Check sheet for the modelled part. Datum: model origin and axes. Units: mm. Face numbers are marked on the shaded views. A direction names the side the tool comes from. Round coordinates to 2 decimals unless told otherwise and drop trailing zeros. Write each loop counter-clockwise with the first axis right and the second up, starting at its lowest first coordinate (ties: lowest second). Pieces come first, ordered by that corner, then holes. Notation, with made-up numbers: (88.25, -35.5) -> (128.25, -35.5) arc R31 ccw to (128.25, 3.5) -> close; hole circle Ø10 at (-11, 47). An arc over 180 degrees is marked (long way). One line per item, written item: value.
Autodesk Inventor part; units mm, degrees
ref_plane "YZ Plane" through (0, 0, 0) normal (1, 0, 0) x (0, 1, 0)
ref_plane "XZ Plane" through (0, 0, 0) normal (0, 1, 0) x (-1, 0, 0)
ref_plane "XY Plane" through (0, 0, 0) normal (0, 0, 1) x (1, 0, 0)
sketch "Sketch1" plane through (0, 0, 0) normal (0, 1, 0) x (-1, 0, 0)
  line L0 (25.9, 0) -> (-25.9, 0)
  line L1 (0, -25.9) -> (0, 25.9)
  circle A0 centre (0, 0) radius 18.5 construction
  circle A1 centre (0, 0) radius 13 construction
  dimension "d0" = 37
  dimension "d1" = 26
sketch "Sketch2" plane through (0, 0, 0) normal (0, 1, 0) x (-1, 0, 0)
  line L0 (77.7, 0) -> (-77.7, 0)
  line L1 (0, -33.3) -> (0, 70.3)
  line L2 (-55.5, 55.5) -> (-55.5, -18.5)
  line L3 (-55.5, -18.5) -> (55.5, -18.5)
  line L4 (55.5, -18.5) -> (55.5, 55.5)
  line L5 (-55.5, 55.5) -> (55.5, 55.5)
  circle A0 centre (0, 37) radius 18.5 construction
  point P0 (0, 0)
  dimension "d3" = 111
  dimension "d29" = 18.5
  dimension "d30" = 55.5
  dimension "d99" = 37
  dimension "d100" = 37
extrude "Extrusion1" add sketch "Sketch2" along normal blind 6
sketch "Sketch6" plane through (0, 0, 0) normal (0, 1, 0) x (-1, 0, 0)
  line L0 (55.5, -18.5) -> (-55.5, -18.5)
  line L1 (55.5, 55.5) -> (55.5, -18.5)
  line L2 (-55.5, -18.5) -> (55.5, -18.5)
  line L3 (55.5, -18.5) -> (55.5, 55.5)
  line L4 (-55.5, 55.5) -> (-55.5, -18.5)
  line L5 (84.7, 0) -> (-84.7, 0)
  line L6 (0, -36.3) -> (0, 70.8)
  arc A0 (-16, 0) -> (16, 0) centre (0, 0) ccw
  line L7 (16, 0) -> (16, 55.5)
  line L8 (55.5, 55.5) -> (-55.5, 55.5)
  line L9 (16, 55.5) -> (55.5, 55.5)
  line L10 (-16, 0) -> (-16, 55.5)
  line L11 (-16, 55.5) -> (-55.5, 55.5)
  point P0 (-17.3617, -21)
  dimension "d18" = 32
extrude "Extrusion5" [suppressed]
sketch "Sketch4" plane through (0, 0, 0) normal (0, 0, 1) x (1, 0, 0)
  line L0 (-18.5, 0) -> (18.5, 0)
  line L1 (18.5, 0) -> (18.5, -2)
  line L2 (18.5, -2) -> (-18.5, -2)
  line L3 (-18.5, -2) -> (-18.5, 0)
  line L4 (-25.9, 0) -> (25.9, 0)
  line L5 (0, -2.4) -> (0, 0.4)
  point P0 (0, 0)
  dimension "d10" = 37
  dimension "d11" = 2
extrude "Extrusion6" [suppressed]
sketch "Sketch5" plane through (0, 0, 0) normal (0, 1, 0) x (-1, 0, 0)
  circle A0 centre (0, 0) radius 18.5 construction
  circle A1 centre (0, 0) radius 18.5 construction
  line L0 (25.9, 0) -> (-25.9, 0)
  line L1 (0, -28.9) -> (0, 26.4)
  line L2 (-18.5, -21) -> (18.5, -21)
  line L3 (18.5, -21) -> (18.5, -18.5)
  line L4 (18.5, -18.5) -> (-18.5, -18.5)
  line L5 (-18.5, -18.5) -> (-18.5, -21)
  dimension "d25" = 37
  dimension "d26" = 21
extrude "Extrusion7" [suppressed]
sketch "Sketch7" plane through (0, 0, 0) normal (0, 0, 1) x (1, 0, 0)
  line L0 (-18.5, 0) -> (18.5, 0)
  line L1 (18.5, 0) -> (18.5, -2)
  line L2 (18.5, -2) -> (-18.5, -2)
  line L3 (-18.5, -2) -> (-18.5, 0)
  line L4 (55.5, 0) -> (-55.5, 0)
  line L5 (-84.7, 0) -> (84.7, 0)
  line L6 (0, -2.4) -> (0, 0.4)
  point P0 (-16, 0)
  point P1 (16, 0)
  dimension "d53" = 2
  dimension "d54" = 18.5
extrude "Extrusion8" [suppressed]
sketch "Sketch8" plane through (0, 0, 0) normal (0, 1, 0) x (-1, 0, 0)
  circle A0 centre (0, 0) radius 12.75
  dimension "d34" = 25.5
extrude "Extrusion9" add sketch "Sketch8" along normal blind 14
pattern_linear "Rectangular Pattern1" count 2 spacing 37 along (0, 0, 1) count 3 spacing 37 along (1, 0, 0) of "Extrusion9" second direction both ways yes
sketch "Sketch9" plane through (0, 6, 0) normal (0, 1, 0) x (1, 0, 0)
  circle A0 centre (0, 0) radius 13
  circle A1 centre (0, 0) radius 15
  dimension "d40" = 26
  dimension "d41" = 30
extrude "Extrusion10" [suppressed]
sketch "Sketch10" plane through (0, 5, 0) normal (0, 1, 0) x (1, 0, 0)
  arc A0 (16, 0) -> (-16, 0) centre (0, 0) ccw
  line L0 (1.5, -18) -> (-1.5, -18)
  line L1 (-29.4, 0) -> (29.4, 0)
  line L2 (0, 36.3) -> (0, -70.8)
  line L3 (1.5, -12) -> (-1.5, -12)
  line L4 (1.5, -12) -> (1.5, -18)
  line L5 (-1.5, -18) -> (-1.5, -12)
  dimension "d48" = 3
  dimension "d49" = 12
  dimension "d50" = 6
extrude "Extrusion11" [suppressed]
fillet "Fillet1" [suppressed]
sketch "Sketch11" plane through (0, 0, 0) normal (0, 1, 0) x (-1, 0, 0)
  line L0 (-60.5, -21) -> (60.5, -21)
  line L1 (60.5, -21) -> (60.5, -47)
  line L2 (60.5, -47) -> (-60.5, -47)
  line L3 (-60.5, -47) -> (-60.5, -21)
  line L4 (84.7, 0) -> (-84.7, 0)
  line L5 (0, -60.1) -> (0, 31.6)
  point P0 (0, 0)
  dimension "d57" = 26
  dimension "d58" = 21
  dimension "d59" = 121
extrude "Extrusion12" [suppressed]
sketch "Sketch12" plane through (0, 0, 0) normal (1, 0, 0) x (0, 1, 0)
  line L0 (6, 55.5) -> (6, -18.5)
  arc A0 (6, -16.5081) -> (5.7334, -47) centre (34, -32) ccw
  line L1 (-6.8, 0) -> (40.8, 0)
  line L2 (0, -67.5) -> (0, 76)
  line L3 (6, -16.5081) -> (6, -47)
  line L4 (6, -47) -> (5.7334, -47)
  line L5 (0, -47) -> (6, -47)
  point P0 (0, 0)
  point P1 (6, 48)
  dimension "d62" = 32
  dimension "d63" = 32
  dimension "d64" = 34
extrude "Extrusion13" [suppressed]
fillet "Fillet3" [suppressed]
sketch "Sketch13" plane through (0, 0, 0) normal (0, 1, 0) x (-1, 0, 0)
  line L0 (84.7, 0) -> (-84.7, 0)
  line L1 (0, -67.5) -> (0, 76)
  line L2 (55.5, 55.5) -> (55.5, -18.5)
  arc A0 (13.0815, 23.9185) -> (13.0815, 13.0815) centre (18.5, 18.5) ccw
  line L3 (-55.5, 55.5) -> (-55.5, -18.5)
  arc A1 (-13.0815, 13.0815) -> (-13.0815, 23.9185) centre (-18.5, 18.5) ccw
  line L4 (18.5, 37) -> (18.5, 0)
  line L5 (-18.5, 0) -> (-18.5, 37)
  line L6 (18.5, 37) -> (18.5, 55.5)
  line L7 (-55.5, 55.5) -> (55.5, 55.5)
  line L8 (-18.5, 55.5) -> (-18.5, 37)
  arc A2 (-9.2871, 53) -> (-13.0815, 23.9185) centre (0, 37) ccw
  arc A3 (13.0815, 23.9185) -> (9.2871, 53) centre (0, 37) ccw
  arc A4 (-13.0815, 13.0815) -> (-18.5, 0) centre (0, 0) ccw
  arc A5 (18.5, 0) -> (13.0815, 13.0815) centre (0, 0) ccw
  point P0 (60.5, -39.254)
  point P1 (-55.5, 48)
  point P2 (-60.5, -16.5081)
  point P3 (-60.5, -47)
  point P4 (55.5, -18.5)
  point P5 (-55.5, -18.5)
  dimension "d68" = 37
  dimension "d71" = 18.5
  dimension "d72" = 18.5
  dimension "d73" = 7.663
  dimension "d74" = 7.663
  dimension "d75" = 18.5
  dimension "d76" = 18.5
  dimension "d77" = 18.5
  dimension "d78" = 18.5
extrude "Extrusion14" [suppressed]
sketch "Sketch14" plane through (0, 0, 0) normal (0, 1, 0) x (-1, 0, 0)
  circle A0 centre (18.5, 18.5) radius 10
  line L0 (39.9, 0) -> (-39.9, 0)
  line L1 (0, -27.9) -> (0, 37.9)
  circle A1 centre (-18.5, 18.5) radius 10
  point P0 (0, 0)
  dimension "d84" = 18.5
  dimension "d85" = 18.5
  dimension "d86" = 20
  dimension "d89" = 37
extrude "Extrusion15" cut sketch "Sketch14" along normal through all
fillet "Fillet4" radius 3 2 edges at (-8.5, 6, 18.5) (28.5, 6, 18.5)
fillet "Fillet5" radius 8 4 edges at (-55.5, 3, 55.5) (55.5, 3, 55.5) (-55.5, 3, -18.5) (55.5, 3, -18.5)
fillet "Fillet6" radius 5 5 edges at (53.1569, 6, 53.1569) (55.5, 6, 18.5) (-53.1569, 6, 53.1569) (-55.5, 6, 18.5) (0, 6, 55.5)
equation "\"d85\" = d84"
properties part number "NespressoSpeedfiller-6X-long-tamper"
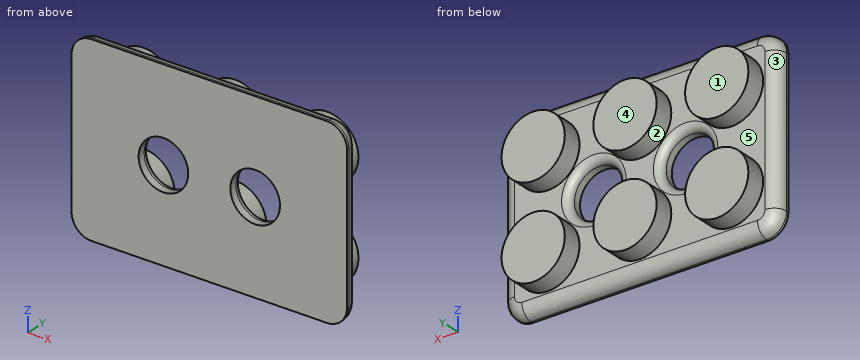
Item 1: Sectioned sample at B-B on x = -18.5. Enter the section's corners in (y, z), and give its area (3 significant figures).
Answer:
outline: (0, -18.5) -> (1, -18.5) arc R5 ccw to (6, -13.5) -> (6, 5.5) arc R3 ccw to (3, 8.5) -> (0, 8.5) -> close; (0, 28.5) -> (3, 28.5) arc R3 ccw to (6, 31.5) -> (6, 50.5) arc R5 ccw to (1, 55.5) -> (0, 55.5) -> close
area: 309 mm^2
Item 2: Sectioned sample at C-C on y = 9.25. Enter the section's corners in (x, z), and give its area (3 significant figures).
Answer:
outline: circle Ø25.5 at (-37, 0); circle Ø25.5 at (-37, 37); circle Ø25.5 at (0, 0); circle Ø25.5 at (0, 37); circle Ø25.5 at (37, 0); circle Ø25.5 at (37, 37)
area: 3,060 mm^2
Item 3: Sectioned sample at A-A on z = 18.5. Enter the section's corners in (x, y).
Answer:
outline: (-55.5, 0) -> (-28.5, 0) -> (-28.5, 3) arc R3 ccw to (-31.5, 6) -> (-50.5, 6) arc R5 ccw to (-55.5, 1) -> close; (-8.5, 0) -> (8.5, 0) -> (8.5, 3) arc R3 ccw to (5.5, 6) -> (-5.5, 6) arc R3 ccw to (-8.5, 3) -> close; (28.5, 0) -> (55.5, 0) -> (55.5, 1) arc R5 ccw to (50.5, 6) -> (31.5, 6) arc R3 ccw to (28.5, 3) -> close
Item 4: Thickness scan on line 1 (X direction, y = 0.95, z = 18.5); line 2 (X direction, y = 8.5, z = 0); line 3 (Z direction, x = -36.5, y = 10.5). Record the ranges inside material, lowest first.
Answer:
line 1: x = -55.5 to -28.5, -8.5 to 8.5, 28.5 to 55.5
line 2: x = -49.75 to -24.25, -12.75 to 12.75, 24.25 to 49.75
line 3: z = -12.74 to 12.74, 24.26 to 49.74
Item 5: Mould release check, pull along X, two halves, no side actions. Record for the marked faces 3, 4 and 5: pulls with the +X half, pulls with the -X half, needs draft (parallel to the pull), parting line crosses it, or undercut.
Answer:
face 3: pulls with the -X half
face 4: needs draft
face 5: undercut
Item 6: Tool access check on the marked faces 1 and 2. Record the directions out of +Z, -Z, +X, -X, +Y, -Y that give a thin tool (end or side, any length) a straight path to the whole face; none if there is none.
Answer:
face 1: +Z, -Z, +X, -X, +Y
face 2: +Y
Item 7: Depth check by flat-ended pin: P1, Ø2, axis at y = 8, z = 45.5, coming from the -X side; P2, Ø5, axis at x = 30.5, z = 20.5, coming from the +Y side; P3, Ø12, axis at x = -18.5, z = 18.5, coming from the -Y side. Enter the tip coordinate at first touch or a pass-through.
Answer:
P1: stops at x = -47.31
P2: stops at y = 6
P3: passes through
Item 8: Sectioned sample at D-D on z = 0. Enter the section's corners in (x, y).
Answer:
outline: (-55.5, 0) -> (55.5, 0) -> (55.5, 1) arc R5 ccw to (50.5, 6) -> (49.75, 6) -> (49.75, 14) -> (24.25, 14) -> (24.25, 6) -> (12.75, 6) -> (12.75, 14) -> (-12.75, 14) -> (-12.75, 6) -> (-24.25, 6) -> (-24.25, 14) -> (-49.75, 14) -> (-49.75, 6) -> (-50.5, 6) arc R5 ccw to (-55.5, 1) -> close
